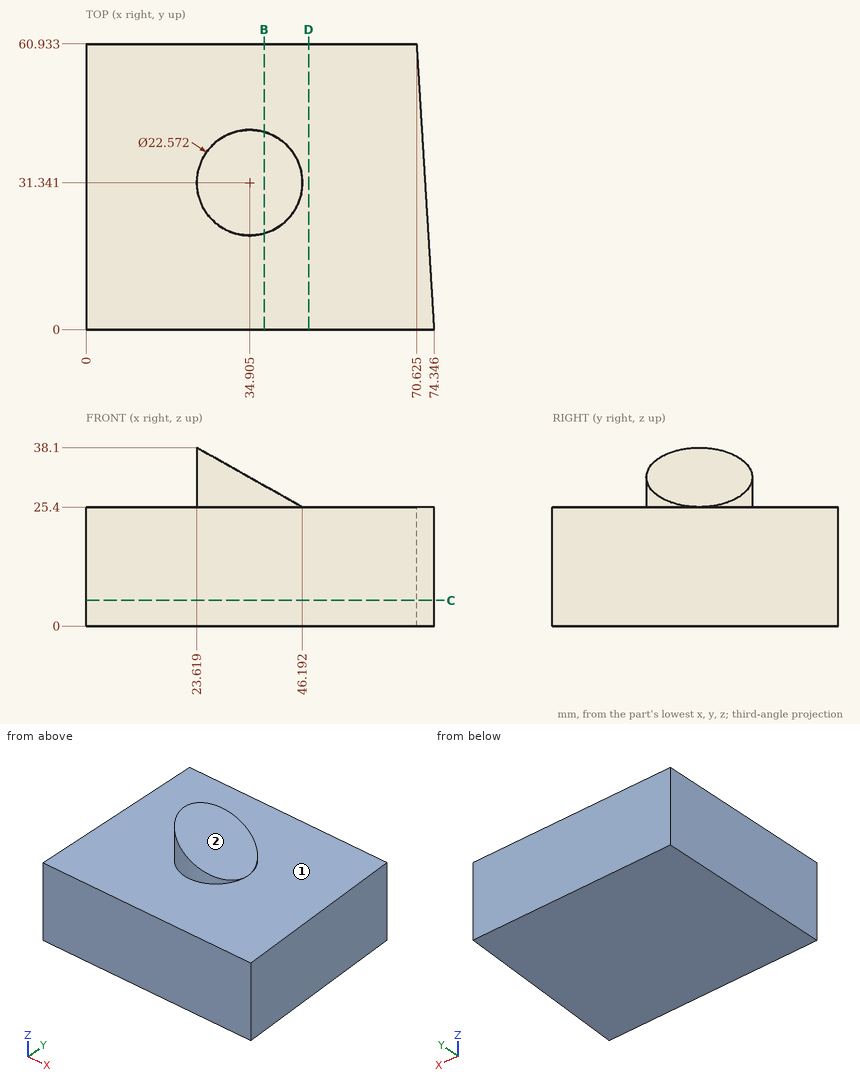
Geometry: see drawing. Coordinates: mm, zero at the bounding-box minimum. A direction names the side the tool comes from. Round coordinates to 2 decimals unless told otherwise and drop trailing zeros. Loops run counter-clockwise (first coordinate to the right, second up) from the corner with the lowest first, then second, coordinate; pieces in that order, holes last. Notation, with made-up numbers: (11, 73) - (35, 73) arc R16 cw to (35, 97) - close; hole circle Ø1 at (-25, 85). An arc over 180 degrees is marked (long way). Use CSV: the item, a comma, the result in double quotes.
Q1. Section query B-B, the plane x = 38. Output: boundary loops of the cut face in (y, z) (1 decimal).
Reported:
outline,"(0, 0) - (60.9, 0) - (60.9, 25.4) - (42.2, 25.4) - (42.2, 30) - (20.5, 30) - (20.5, 25.4) - (0, 25.4) - close"
Q2. Ray query, line 1 along Z through (x, y) = (22.5, 48); line 2 along X through (y, z) = (15, 21); line 3 along X through (y, z) = (19, 4.5) (1 decimal). Return the intervals inside material, ascending.
Reported:
line 1,"0 to 25.4"
line 2,"0 to 73.43"
line 3,"0 to 73.2"
Q3. Reachability of the marked faces 1 and 2 from +Z, -Z, +X, -X, +Y, -Y: full face, straight path, thin tool, end or side. Return the list, or none.
Reported:
face 1,"+Z"
face 2,"+Z, +X, +Y, -Y"
Q4. Section query D-D, the plane x = 47.5. Output: boundary loops of the cut face in (y, z).
Reported:
outline,"(0, 0) - (60.93, 0) - (60.93, 25.4) - (0, 25.4) - close"
Q5. Pin query (flat end, axial travel): pin 1 Ø4 at (y, z) = (17.5, 24.5) entering from +X; pin 2 Ø2 at (x, y) = (12.5, 18) entering from +Z. Return the tip coordinate at first contact, or that it passes through.
Reported:
pin 1,"x = 73.4"
pin 2,"z = 25.4"
Q6. Section query C-C, the plane z = 5.5. Output: boundary loops of the cut face in (x, y) (1 decimal).
Reported:
outline,"(0, 0) - (74.3, 0) - (70.6, 60.9) - (0, 60.9) - close"
